Design review of the part built by this model. Coordinates are the model's own, in mm. A direction names the side the tool comes from. Coordinates: 2 decimals unless noted, no trailing zeros. Loops run counter-clockwise (first coordinate to the right, second up) from the corner with the lowest first, then second, coordinate; pieces in that order, holes last. Notation, with made-up numbers: (15.5, 23.5) -> (47.5, 23.5) arc R10 ccw to (47.5, 39.5) -> close; hole circle Ø9 at (60, 65.25). An arc over 180 degrees is marked (long way). Use one line per item in the form item = value. Start each with the question number.
1. For pin 1 (4 mm diameter, centred on y = 1, z = -6, fed in from -X); pin 2 (2 mm diameter, centred on x = -8, z = -2, fed in from -Y); pin 3 (9 mm diameter, centred on x = 0, y = 0, fed in from +Z); pin 4 (6 mm diameter, centred on y = 1.5, z = -6.5, fed in from +X), all flat-tipped, find the tip position at first contact; note any pin that passes through.
2. Wall thickness on line 1 (X direction, y = 0, z = -7); line 2 (Y direction, x = 0, z = -10.65); line 3 (Y direction, x = 0, z = -7): over which ranges is each line inside the solid? List them lowest first. Write a range as from..to.
3. Machinability: for faces 1 (the face through (-9.615, -0.026, -8.572)), 2 (the face through (6, 0, -4.762)), 3 (the face through (13, 4, 0)), which of the approach directions +Z, -Z, +X, -X, +Y, -Y give a long, thin tool a straight path to every point of the face, cutting with its end or side? Answer none if there is none.
4. Consider section A-A (x = 0). State the section outline as (y, z) points, then the cut area to 3 significant figures.
5. Consider section C-C (y = -5.75). State the section outline as (x, z) points, then the cut area to 3 significant figures.
6. The part is to be moulded in two halves that separate along X. For faces 4 (the face through (13.67, 4.3, -6.2)), 5 (the face through (0, 0, -11.697)), 6 (the face through (0, 0, -12.586)), say which applies: released by +X, released by -X, zero draft, split by the parting line, or undercut.
7. Consider section D-D (z = -3). State the section outline as (x, y) points, then the cut area to 3 significant figures.
8. Consider section B-B (z = -5.25). State the section outline as (x, y) points (1 decimal), then the cut area to 3 significant figures.
from build123d import *

# Parameters (mm, degrees)
F3_DEPTH = 25.4
F5_D     = 2.2606
F5_DEPTH = 5.715
F5_TIP   = 0.6791527577


with BuildPart() as f1:
    # F0 (on Front) → F1 (revolve)
    with BuildSketch(Plane.XZ):
        Polygon((14.330415332, -12.5857), (14.330415332, 0), (13.314415332, 0), (13.314415332, -4.7625), (5.1689, -4.7625), (5.1689, -8.8265), (4.0005, -8.8265), (4.0005, -11.6967), (0, -11.6967), (0, -12.5857), align=None)
    revolve(axis=Axis((0, 0, -12.1412), (0, 0, 1)))

    # F2 (on Right) → F3 (cut)
    with BuildSketch(Plane.YZ):
        with BuildLine():
            Line((-1.190625, 0), (-1.190625, -7.381875))
            ThreePointArc((-1.190625, -7.381875), (0, -8.5725), (1.190625, -7.381875))
            Line((1.190625, -7.381875), (1.190625, 0))
            Line((1.190625, 0), (-1.190625, 0))
        make_face()
    extrude(amount=-F3_DEPTH, mode=Mode.SUBTRACT)

    # F5
    with Locations(Plane.XY.offset(-4.7625)):
        with Locations((9.525, 0), (-4.7625, 8.248891971), (-4.7625, -8.248891971)):
            Hole(F5_D / 2, depth=F5_DEPTH)
            with Locations((0, 0, -(F5_DEPTH + F5_TIP / 2))):  # 118° drill point
                Cone(0, F5_D / 2, F5_TIP, mode=Mode.SUBTRACT)


solid = f1.part
Geometry check:
q1.pin_1 = -14.29
q1.pin_2 = -12.5
q1.pin_3 = -8.83
q1.pin_4 = 14.33
q2.line_1 = 5.17..8.39, 10.66..14.33
q2.line_2 = -14.33..-4, 4..14.33
q2.line_3 = -14.33..-5.17, 5.17..14.33
q3.face_1 = +Z, -X
q3.face_2 = +Z
q3.face_3 = +Z, +X, -X, +Y, -Y
q4.outline = (-14.33, -12.59) -> (14.33, -12.59) -> (14.33, 0) -> (13.31, 0) -> (13.31, -4.76) -> (5.17, -4.76) -> (5.17, -8.83) -> (4, -8.83) -> (4, -11.7) -> (-4, -11.7) -> (-4, -8.83) -> (-5.17, -8.83) -> (-5.17, -4.76) -> (-13.31, -4.76) -> (-13.31, 0) -> (-14.33, 0) -> close
q4.area = 169 mm²
q5.outline = (-13.13, -12.59) -> (13.13, -12.59) -> (13.13, 0) -> (12.01, 0) -> (12.01, -4.76) -> (-12.01, -4.76) -> (-12.01, 0) -> (-13.13, 0) -> close
q5.area = 216 mm²
q6.face_4 = split by the parting line
q6.face_5 = undercut
q6.face_6 = zero draft
q7.outline = (-14.28, -1.19) arc R14.33 ccw (long way) to (-14.28, 1.19) -> (-13.26, 1.19) arc R13.31 cw (long way) to (-13.26, -1.19) -> close
q7.area = 85.8 mm²
q8.outline = (-14.3, -1.2) arc R14.3 ccw (long way) to (-14.3, 1.2) -> (-5, 1.2) arc R5.2 cw (long way) to (-5, -1.2) -> close; hole circle Ø2.3 at (-4.8, -8.2); hole circle Ø2.3 at (-4.8, 8.2); hole circle Ø2.3 at (9.5, 0)
q8.area = 527 mm²
